Source: three-view drawing plus pictorial views. Frame: mm from the lowest corner of the part. Coordinates: 2 decimals unless noted, no trailing zeros. Write each loop counter-clockwise with the first axis right and the second up, starting at its lowest first coordinate (ties: lowest second). Pieces come first, ordered by that corner, then holes. Notation, with made-up numbers: M -14.75,26.5 L 24.25,26.5 A25 cw 24.25,62.5 Z; hole C -33.75,16 d2. An arc over 180 degrees is marked long. Use CSV: the item, a comma, the result in double quotes.
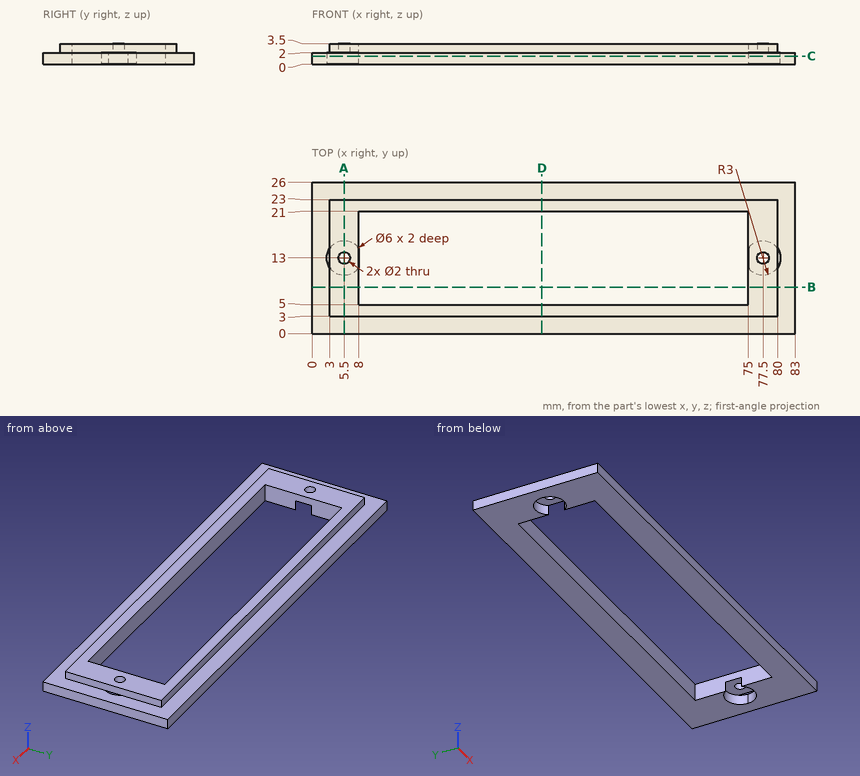
1. Contact query for flat-ended pins moving along their axis: pin 1 Ø0.8 at (x, z) = (29.5, 3) entering from -Y; pin 2 Ø1.5 at (x, y) = (4.5, 12) entering from -Z; pin 3 Ø1.2 at (x, y) = (77.5, 13) entering from -Z; pin 4 Ø1.2 at (y, z) = (10, 3) entering from -X. Output: stop coordinate, or through.
Resolved:
pin 1,"stops at y = 3"
pin 2,"stops at z = 2"
pin 3,"passes through"
pin 4,"stops at x = 3"
2. Section A-A (x = 5.5). Return loops of the section in (y, z).
Resolved:
outline,"M 0,0 L 10,0 L 10,2 L 12,2 L 12,3.5 L 3,3.5 L 3,2 L 0,2 Z; M 14,2 L 16,2 L 16,0 L 26,0 L 26,2 L 23,2 L 23,3.5 L 14,3.5 Z"
3. Section B-B (y = 8). Return loops of the section in (x, z), then the cut area to 3 significant figures.
Resolved:
outline,"M 0,0 L 8,0 L 8,3.5 L 3,3.5 L 3,2 L 0,2 Z; M 75,0 L 83,0 L 83,2 L 80,2 L 80,3.5 L 75,3.5 Z"
area,"47.0 mm^2"
4. Section D-D (x = 39.5). Return loops of the section in (y, z).
Resolved:
outline,"M 0,0 L 5,0 L 5,3.5 L 3,3.5 L 3,2 L 0,2 Z; M 21,0 L 26,0 L 26,2 L 23,2 L 23,3.5 L 21,3.5 Z"
5. Section C-C (z = 1.4). Return loops of the section in (x, y).
Resolved:
outline,"M 0,0 L 83,0 L 83,26 L 0,26 Z; hole M 8,5 L 75,5 L 75,11.34 A3 ccw long 75,14.66 L 75,21 L 8,21 L 8,14.66 A3 ccw long 8,11.34 Z"
6. Material intervals for line 1 (X direction, y = 13, z = 2.7); line 2 (Y direction, x = 61.5, z = 0.7); line 3 (Y direction, x = 16.5, z = 3.15), sorted ascending. Write a range as [from, to].
Resolved:
line 1,"x = [3, 4.5], [6.5, 8], [75, 76.5], [78.5, 80]"
line 2,"y = [0, 5], [21, 26]"
line 3,"y = [3, 5], [21, 23]"
